from build123d import *

# Parameters (mm, degrees)
F0_R     = 27.9704951592
F0_R_2   = 22.0413133634
F1_DEPTH = 76.2
F3_DEPTH = 12.7
F5_R     = 6.35
F6_R     = 4.2845599963
F7_DEPTH = 25.4
F8_DEPTH = 25.4


# Not quite as in the source:
# - a fillet or chamfer that OpenCascade refuses, or shapes differently, is made with other operations: its cross-section is extruded or revolved along the edge and cut away or added


with BuildPart() as f1:
    # F0 (on Top) → F1 (new body)
    with BuildSketch(Plane.XY):
        Circle(F0_R)
        Circle(F0_R_2, mode=Mode.SUBTRACT)
    extrude(amount=F1_DEPTH)

    # F2 (on face) → F3 (join)
    with BuildSketch(Plane.XY.offset(76.2)):
        with BuildLine():
            Line((-54.7763327301, -37.8764942288), (54.7763327301, -37.8764942288))
            ThreePointArc((54.7763327301, -37.8764942288), (59.2664607906, -36.0166222894), (61.1263327301, -31.5264942288))
            Line((61.1263327301, -31.5264942288), (61.1263327301, 31.5264942288))
            ThreePointArc((61.1263327301, 31.5264942288), (59.2664607906, 36.0166222894), (54.7763327301, 37.8764942288))
            Line((54.7763327301, 37.8764942288), (-54.7763327301, 37.8764942288))
            ThreePointArc((-54.7763327301, 37.8764942288), (-59.2664607906, 36.0166222894), (-61.1263327301, 31.5264942288))
            Line((-61.1263327301, 31.5264942288), (-61.1263327301, -31.5264942288))
            ThreePointArc((-61.1263327301, -31.5264942288), (-59.2664607906, -36.0166222894), (-54.7763327301, -37.8764942288))
        make_face()
    extrude(amount=F3_DEPTH)

    # F4: fillet of radius 7.62 on 1 edges, made by hand

    # F4_s1 → F4_t2 (revolve, cut)
    with BuildSketch(Plane.XZ):
        with BuildLine():
            ThreePointArc((27.9704951592, 7.4300426513), (26.3065187789, 2.6771295823), (22.0413133634, 0))
            Line((22.0413133634, 0), (27.9704951592, 0))
            Line((27.9704951592, 0), (27.9704951592, 7.4300426513))
        make_face()
    revolve(axis=Axis((0, 0, 0), (0, 0, 1)), mode=Mode.SUBTRACT)

    # F5
    f5_edges = [f1.edges().sort_by_distance(p)[0] for p in [
        (-61.126333, 0, 76.2),
        (0, -37.876494, 76.2),
        (61.126333, 0, 76.2),
        (0, 37.876494, 76.2),
        (-59.266461, -36.016622, 76.2),
        (59.266461, -36.016622, 76.2),
        (-59.266461, 36.016622, 76.2),
        (59.266461, 36.016622, 76.2),
    ]]
    fillet(f5_edges, radius=F5_R)

    # F6 (on face) → F7 (cut)
    with BuildSketch(Plane(origin=(0, 0, 76.2), x_dir=(1, 0, 0), z_dir=(0, 0, -1))):
        with Locations((46.7646792531, -23.6378517002)):
            Circle(F6_R)
        with Locations((-46.7646792531, -23.6378517002)):
            Circle(F6_R)
        with Locations((46.7646792531, 23.6378517002)):
            Circle(F6_R)
        with Locations((-46.7646792531, 23.6378517002)):
            Circle(F6_R)
    extrude(amount=-F7_DEPTH, mode=Mode.SUBTRACT)

    # F8 (cut): a face of the model
    f8_faces = [f1.faces().sort_by_distance(p)[0] for p in [
        (0, 0, 76.2),
    ]]
    extrude(f8_faces, amount=-F8_DEPTH, mode=Mode.SUBTRACT)


solid = f1.part
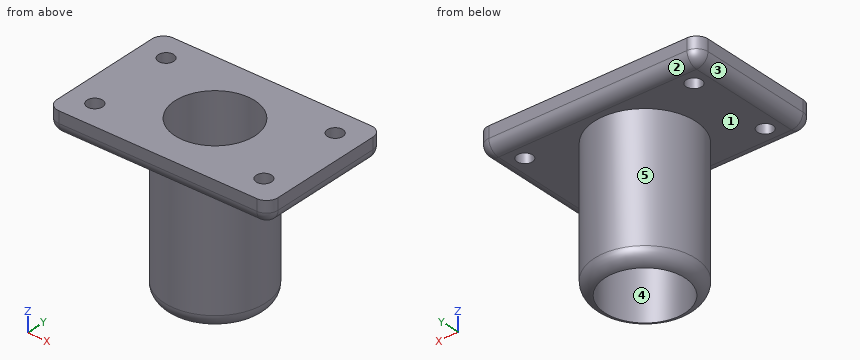
CAD build for the part. Positions are in the model's coordinates, mm. Face numbers are marked on the shaded views. A direction names the side the tool comes from. Round coordinates to 2 decimals unless told otherwise and drop trailing zeros. Loops run counter-clockwise (first coordinate to the right, second up) from the corner with the lowest first, then second, coordinate; pieces in that order, holes last.
(1) Cut at A-A (x = 0). Give the cut face in (y, z).
(2) Two-plate mould, pull along X, no slides. Class the marked faces 3, 4 and 5: +X half, -X half, draft (parallel to the pull), parting line (faces both ways), or undercut.
(3) Cut at C-C (x = -31.5). Give the cut face in (y, z).
(4) Cut at B-B (y = 0). Give the cut face in (x, z), plus the area to 3 significant figures.
(5) Which spindle directions (+Z, -Z, +X, -X, +Y, -Y) get a long thin tool onto all of the face, cutting with end or side? Do the marked faces 1 and 2. Say none if no direction does.
(6) Cut at D-D (z = 43.5). Give the cut face in (x, y).
(7) Wall check: line 1 along Y through (x, z) = (0, 35); line 2 along Z through (x, y) = (22.5, 28.5); line 3 along Y through (x, z) = (12.5, 46.5). Give the ranges that are in metal, low to high.
(8) Drop flat-ended pins along their axis: pin 1 (3 mm diameter, centred on x = -3.5, z = 71.5, fed in from +Y); pin 2 (12 mm diameter, centred on y = -17.5, z = 41, fed in from +X); pin 3 (7.5 mm diameter, centred on x = -46.76, y = 23.64, fed in from +Z); pin 4 (2 mm diameter, centred on y = 1.5, z = 50.5, fed in from +X). Give the stop position or say it passes through.
Findings below:
1. outline: (-37.88, 82.55) arc R6.35 ccw to (-31.53, 76.2) - (-27.97, 76.2) - (-27.97, 7.43) arc R7.62 ccw to (-22.04, 0) - (-22.04, 88.9) - (-37.88, 88.9) - close; (22.04, 0) arc R7.62 ccw to (27.97, 7.43) - (27.97, 76.2) - (31.53, 76.2) arc R6.35 ccw to (37.88, 82.55) - (37.88, 88.9) - (22.04, 88.9) - close
2. face 3: -X half
2. face 4: undercut
2. face 5: parting line
3. outline: (-37.88, 82.55) arc R6.35 ccw to (-31.53, 76.2) - (31.53, 76.2) arc R6.35 ccw to (37.88, 82.55) - (37.88, 88.9) - (-37.88, 88.9) - close
4. outline: (-61.13, 82.55) arc R6.35 ccw to (-54.78, 76.2) - (-27.97, 76.2) - (-27.97, 7.43) arc R7.62 ccw to (-22.04, 0) - (-22.04, 88.9) - (-61.13, 88.9) - close; (22.04, 0) arc R7.62 ccw to (27.97, 7.43) - (27.97, 76.2) - (54.78, 76.2) arc R6.35 ccw to (61.13, 82.55) - (61.13, 88.9) - (22.04, 88.9) - close
4. area: 1,860 mm2
5. face 1: -Z
5. face 2: -Z, +X, -X, +Y
6. outline: circle Ø55.94 at (0, 0); hole circle Ø44.08 at (0, 0)
7. line 1: y = -27.97 to -22.04, 22.04 to 27.97
7. line 2: z = 76.2 to 88.9
7. line 3: y = -25.02 to -18.15, 18.15 to 25.02
8. pin 1: stops at y = 27.9
8. pin 2: stops at x = 25.5
8. pin 3: passes through
8. pin 4: stops at x = 27.97
